Can you work these out from the drawing? Everything is in mm from the part's minimum corner. A direction names the side the tool comes from. Coordinates: 2 decimals unless noted, no trailing zeros. Order: outer loops, then holes, each group sorted by start corner. A loop starts at its lowest first (then second) coordinate and runs counter-clockwise, first axis right, second up. Notation, with made-up numbers: (-35, -16.75) - (-9, -16.75) arc R23 cw to (-9, 11.25) - close; hole circle Ø4 at (-31, -33). An arc over 180 degrees is marked (long way). Answer as CSV lines item,"result". Start each with the question number.
Q1. For the marked faces 1 and 2, which set-ups out of +Z, -Z, +X, -X, +Y, -Y let a thin tool reach every point of the face, with its end or its side?
Q2. I need wall thicknesses on line 1 (Z direction, x = 2.5, y = 18); line 2 (Y direction, x = 7, z = 7.5). Which ranges of each line are inside material? Lowest first, please.
Q3. Suppose I cut it at D-D (y = 3.5). Please give me the cut outline in (x, z), then the cut area to 3 significant figures.
Q4. For pin 1 Ø5.5 at (x, z) = (13, 5) entering from +Y; pin 2 Ø3 at (y, z) = (10, 6.5) entering from +X, each with a flat end and sliding along its axis, tell me the tip position at first contact or that it passes through.
Q5. Thinking about a two-plate mould opening in X: for the marked faces 3, 4 and 5, which applies, released by +X, released by -X, zero draft, split by the parting line, or undercut?
Q6. Suppose I cut it at A-A (y = 18). Please give me the cut outline in (x, z), then the cut area to 3 significant figures.
Q7. Suppose I cut it at B-B (z = 5). Please give me the cut outline in (x, y).
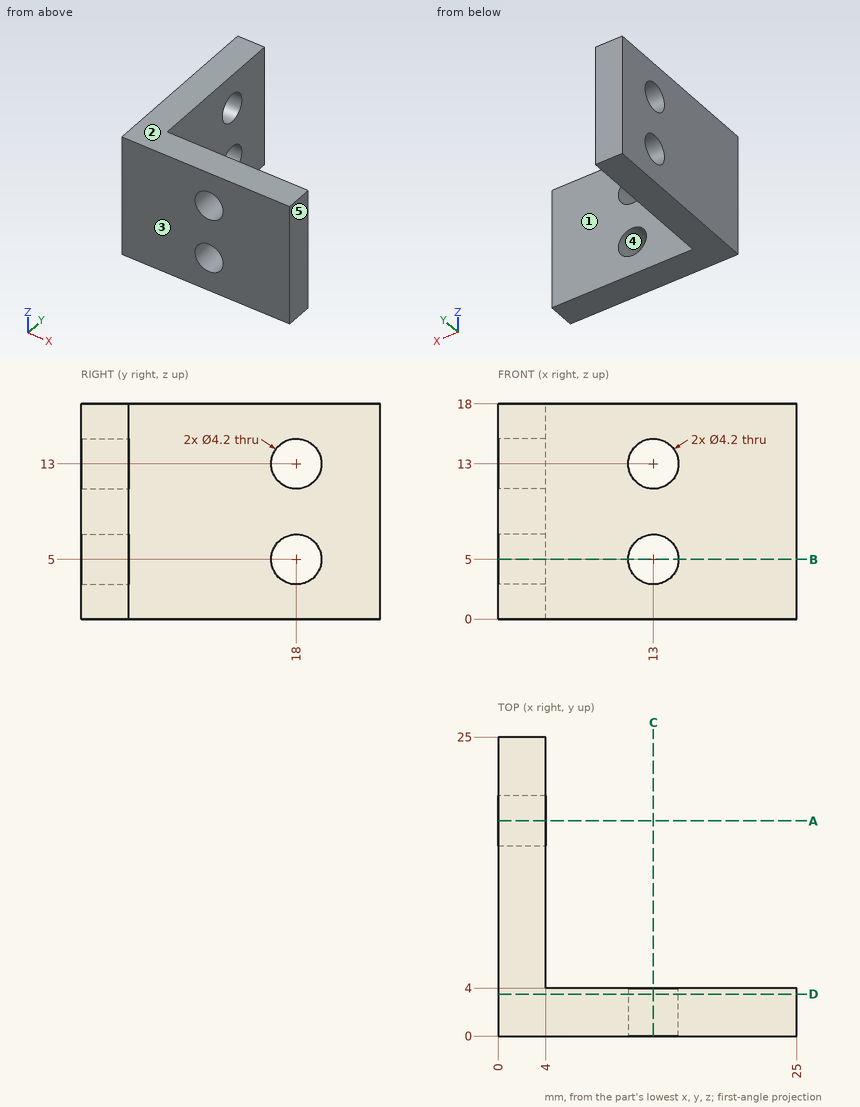
Here are the results:
1,face 1,"+Z, -Z, +X, +Y"
1,face 2,"+Z, +X, -X, +Y, -Y"
2,line 1,"z = 0 to 2.9, 7.1 to 10.9, 15.1 to 18"
2,line 2,"y = 0 to 4"
3,outline,"(0, 0) - (25, 0) - (25, 18) - (0, 18) - close; hole circle Ø4.2 at (13, 5); hole circle Ø4.2 at (13, 13)"
3,area,"422 mm²"
4,pin 1,"stops at y = 4"
4,pin 2,"stops at x = 4"
5,face 3,"zero draft"
5,face 4,"undercut"
5,face 5,"released by +X"
6,outline,"(0, 0) - (4, 0) - (4, 2.9) - (0, 2.9) - close; (0, 7.1) - (4, 7.1) - (4, 10.9) - (0, 10.9) - close; (0, 15.1) - (4, 15.1) - (4, 18) - (0, 18) - close"
6,area,"38.4 mm²"
7,outline,"(0, 0) - (10.9, 0) - (10.9, 4) - (4, 4) - (4, 15.9) - (0, 15.9) - close; (0, 20.1) - (4, 20.1) - (4, 25) - (0, 25) - close; (15.1, 0) - (25, 0) - (25, 4) - (15.1, 4) - close"
